```python
from build123d import *

# Parameters (mm, degrees)
SKETCH_1_R      = 3
EXTRUDE_1_DEPTH = 12
SKETCH_2_R      = 6.5
EXTRUDE_2_DEPTH = 8
CHAMFER_1_SIZE  = 0.5


with BuildPart() as part:
    # 草图1 → 凸台-拉伸1 (new body)
    with BuildSketch(Plane(origin=(0, 0, 0), x_dir=(0, 0, -1), z_dir=(1, 0, 0))):
        Circle(SKETCH_1_R)
    extrude(amount=EXTRUDE_1_DEPTH)

    # 草图2 → 凸台-拉伸2 (add)
    with BuildSketch(Plane(origin=(12, 0, 0), x_dir=(0, 0, -1), z_dir=(1, 0, 0))):
        Circle(SKETCH_2_R)
    extrude(amount=EXTRUDE_2_DEPTH)

    # 草图3 → 旋转2 (revolve)
    with BuildSketch(Plane(origin=(0, 0, 0), x_dir=(1, 0, 0), z_dir=(0, 1, 0))):
        with BuildLine():
            Line((15, 0), (23, 0))
            ThreePointArc((23, 0), (22.337104701, 2.20538709), (20.568133892, 3.679803812))
            Line((20.568133892, 3.679803812), (20.568133892, 4.110994158))
            Line((20.568133892, 4.110994158), (20, 4.650865374))
            Line((20, 4.650865374), (20, 3.872983346))
            ThreePointArc((20, 3.872983346), (16.550510257, 3.16227766), (15, 0))
        make_face()
    revolve(axis=Axis((15, 0, 0), (1, 0, 0)))

    # 倒角1
    chamfer_1_edges = [part.edges().sort_by_distance(p)[0] for p in [
        (0, 0, 3),
    ]]
    chamfer(chamfer_1_edges, length=CHAMFER_1_SIZE)


solid = part.part
```
Verification items for the finished model (mm, model axes). A direction names the side the tool comes from. Give positions to 0.01 mm unless a question says otherwise; leave off trailing zeros. Order: outer loops, then holes, each group sorted by start corner. A loop starts at its lowest first (then second) coordinate and runs counter-clockwise, first axis right, second up. Notation, with made-up numbers: (-21, 30.5) -> (2, 30.5) arc R37 cw to (2, 68.5) -> close; hole circle Ø10 at (-29, 25). An arc over 180 degrees is marked (long way). One line per item, written item: value.
(1) Scan lines: line 1 along X through (y, z) = (2.5, -5); line 2 along X through (y, z) = (1, 3.75); line 3 along Y through (x, z) = (12.5, 5). Record each from-to range of solid material in increasing order. Write a range as [from, to].
Final values:
line 1: [12, 20]
line 2: [12, 20.57]
line 3: [-4.15, 4.15]
(2) Sectioned sample at D-D on x = 2.25. Record the cut outline in (y, z).
Final values:
outline: circle Ø6 at (0, 0)
(3) Gauge pin test, flat ends, axial feed: pin 1 (6 mm diameter, centred on y = -3.5, z = -5, fed in from +X); pin 2 (1.5 mm diameter, centred on x = 20, z = 4, fed in from -Y); pin 3 (4 mm diameter, centred on y = 0.5, z = 2.5, fed in from -X); pin 4 (1 mm diameter, centred on x = 8.5, z = -4.5, fed in from -Y). Record the tip position at first contact, or that the pin passes through.
Final values:
pin 1: x = 21.52
pin 2: y = -5.63
pin 3: x = 0
pin 4: through
(4) Tool access check on faces 1 (the face through (12, -1, -3)), 2 (the face through (20, -4, -3)), 3 (the face through (15.944, -3.955, 5.158)). Record the directions out of +Z, -Z, +X, -X, +Y, -Y that give a thin tool (end or side, any length) a straight path to the whole face; none if there is none.
Final values:
face 1: -X
face 2: +X
face 3: +X, -X
(5) Sectioned sample at A-A on y = 0. Record the cut outline in (x, z), then the cut area to 3 significant figures.
Final values:
outline: (0, -2.5) -> (0.5, -3) -> (12, -3) -> (12, -6.5) -> (20, -6.5) -> (20, -4.65) -> (20.57, -4.11) -> (20.57, -3.68) arc R4 ccw to (20.57, 3.68) -> (20.57, 4.11) -> (20, 4.65) -> (20, 6.5) -> (12, 6.5) -> (12, 3) -> (0.5, 3) -> (0, 2.5) -> close
area: 194 mm^2
(6) Sectioned sample at C-C on x = 19.5. Record the cut outline in (y, z).
Final values:
outline: circle Ø13 at (0, 0)
